from build123d import *

# Parameters (mm, degrees)
CUT_EXTRUDE1_DEPTH       = 5
CUT_EXTRUDE3_DEPTH       = 45
SKETCH8_R                = 40
CUT_EXTRUDE4_DEPTH       = 32
SKETCH9_R                = 32
SKETCH9_R_2              = 24.5
CUT_EXTRUDE5_DEPTH       = 14
SKETCH10_R               = 26
CUT_EXTRUDE6_DEPTH       = 14
FILLET1_R                = 7
FILLET2_R                = 7
CUT_REVOLVE1_START       = 22
CUT_REVOLVE1_DEPTH       = 30.5
CUT_EXTRUDE12_DEPTH      = 5
SKETCH18_W               = 13
SKETCH18_H               = 8
CUT_EXTRUDE13_DEPTH      = 5
INTERSECT1_OUTLINE_R     = 42
INTERSECT1_DEPTH         = 55
SKETCH20_W               = 6
SKETCH20_H               = 3
BOSS_EXTRUDE1_DEPTH      = 8
BOSS_EXTRUDE2_DEPTH      = 1
BOSS_EXTRUDE2_DEPTH_BACK = 1
SKETCH21_W               = 6
SKETCH21_H               = 6
BOSS_EXTRUDE3_DEPTH      = 7
SKETCH19_R               = 1.5
CUT_EXTRUDE14_DEPTH      = 8
SKETCH23_W               = 20
SKETCH23_H               = 7
CUT_EXTRUDE15_DEPTH      = 7
SKETCH24_W               = 44
SKETCH24_H               = 3.5
CUT_EXTRUDE16_DEPTH      = 5


# Read off the part's stored shape, not the designer's step: Cut-Revolve1, Intersect1
with BuildPart() as part:
    # Sketch1 → Revolve1 (revolve)
    with BuildSketch(Plane.XY, mode=Mode.PRIVATE) as revolve1_sk:
        with BuildLine():
            Line((22.5, 0), (32, 0))
            ThreePointArc((32, 0), (33.414213562, 0.585786438), (34, 2))
            Line((34, 2), (34, 18))
            Line((34, 18), (40, 18))
            ThreePointArc((40, 18), (41.414213562, 18.585786438), (42, 20))
            Line((42, 20), (42, 55))
            ThreePointArc((42, 55), (40.535533906, 58.535533906), (37, 60))
            Line((37, 60), (0, 60))
            Line((0, 60), (0, 18))
            Line((0, 18), (22.5, 18))
            Line((22.5, 18), (22.5, 0))
        make_face()
    revolve(revolve1_sk.sketch.rotate(Axis((0, 2, 0), (0, 1, 0)), 90), axis=Axis((0, 2, 0), (0, 1, 0)))

    # Sketch5 → Cut-Extrude1 (cut)
    with BuildSketch(Plane(origin=(0, 60, 0), x_dir=(1, 0, 0), z_dir=(0, 1, 0))):
        with BuildLine():
            Line((-42, 0), (-40, 0))
            Line((-40, 0), (40, 0))
            Line((40, 0), (42, 0))
            ThreePointArc((42, 0), (0, 42), (-42, 0))
        make_face()
    extrude(amount=-CUT_EXTRUDE1_DEPTH, mode=Mode.SUBTRACT)

    # Sketch7 → Cut-Extrude3 (cut)
    with BuildSketch(Plane.XZ.offset(-18)):
        with BuildLine():
            Line((-21, 0), (21, 0))
            ThreePointArc((21, 0), (0, -21), (-21, 0))
        make_face()
    extrude(amount=-CUT_EXTRUDE3_DEPTH, mode=Mode.SUBTRACT)

    # Sketch8 → Cut-Extrude4 (cut)
    with BuildSketch(Plane(origin=(0, 52.5, 0), x_dir=(1, 0, 0), z_dir=(0, 1, 0))):
        with Locations(Location((0, 0, 0), (0, 0, 270))):
            Circle(SKETCH8_R)
        with BuildLine():
            Line((22.912878475, -2), (-22.912878475, -2))
            ThreePointArc((-22.912878475, -2), (0, 23), (22.912878475, -2))
        make_face(mode=Mode.SUBTRACT)
    extrude(amount=-CUT_EXTRUDE4_DEPTH, mode=Mode.SUBTRACT)

    # Sketch9 → Cut-Extrude5 (cut)
    with BuildSketch(Plane(origin=(0, 2, 0), x_dir=(-1, 0, 0), z_dir=(0, -1, 0))):
        with Locations(Location((0, 0, 0), (0, 0, 90))):
            Circle(SKETCH9_R)
        with Locations(Location((0, 0, 0), (0, 0, 90))):
            Circle(SKETCH9_R_2, mode=Mode.SUBTRACT)
    extrude(amount=-CUT_EXTRUDE5_DEPTH, mode=Mode.SUBTRACT)

    # Sketch10 → Cut-Extrude6 (cut)
    with BuildSketch(Plane(origin=(0, 2, 0), x_dir=(-1, 0, 0), z_dir=(0, -1, 0))):
        Circle(SKETCH10_R)
    extrude(amount=-CUT_EXTRUDE6_DEPTH, mode=Mode.SUBTRACT)

    # Fillet1
    fillet1_edges = [part.edges().sort_by_distance(p)[0] for p in [
        (21, 36.5, 0),
        (-21, 36.5, 0),
    ]]
    fillet(fillet1_edges, radius=FILLET1_R)

    # Fillet2
    fillet2_edges = [part.edges().sort_by_distance(p)[0] for p in [
        (-22.912878475, 36.5, 2),
        (22.912878475, 36.5, 2),
    ]]
    fillet(fillet2_edges, radius=FILLET2_R)

    # Cut-Revolve1 outline → Cut-Revolve1 (cut)
    with BuildSketch(Plane(origin=(0, 0, 0), x_dir=(1, 0, 0), z_dir=(0, 1, 0)).offset(CUT_REVOLVE1_START)):
        with BuildLine():
            Line((-34.641016151, -20), (-36.373066959, -21))
            ThreePointArc((-36.373066959, -21), (0, -42), (36.373066959, -21))
            Line((36.373066959, -21), (34.641016151, -20))
            ThreePointArc((34.641016151, -20), (0, -40), (-34.641016151, -20))
        make_face()
    extrude(amount=CUT_REVOLVE1_DEPTH, mode=Mode.SUBTRACT)

    # Sketch15 → Cut-Extrude12 (cut)
    with BuildSketch(Plane(origin=(0, 20.5, 0), x_dir=(1, 0, 0), z_dir=(0, 1, 0))):
        with BuildLine():
            Line((-28.124355653, -3.514579578), (-26.124355653, -3.514579578))
            ThreePointArc((-26.124355653, -3.514579578), (-24.710142091, -2.928793141), (-24.124355653, -1.514579578))
            Line((-24.124355653, -1.514579578), (-24.124355653, 8.485420422))
            ThreePointArc((-24.124355653, 8.485420422), (-24.710142091, 9.899633984), (-26.124355653, 10.485420422))
            Line((-26.124355653, 10.485420422), (-28.124355653, 10.485420422))
            ThreePointArc((-28.124355653, 10.485420422), (-29.538569215, 9.899633984), (-30.124355653, 8.485420422))
            Line((-30.124355653, 8.485420422), (-30.124355653, -1.514579578))
            ThreePointArc((-30.124355653, -1.514579578), (-29.538569215, -2.928793141), (-28.124355653, -3.514579578))
        make_face()
    extrude(amount=-CUT_EXTRUDE12_DEPTH, mode=Mode.SUBTRACT)

    # Sketch18 → Cut-Extrude13 (cut)
    with BuildSketch(Plane(origin=(0, 55, 0), x_dir=(1, 0, 0), z_dir=(0, 1, 0))):
        with Locations((0.796512215, 32.951769165)):
            Rectangle(SKETCH18_W, SKETCH18_H)
    extrude(amount=-CUT_EXTRUDE13_DEPTH, mode=Mode.SUBTRACT)

    # Intersect1 outline → Intersect1 (cut)
    with BuildSketch(Plane(origin=(0, 0, 0), x_dir=(1, 0, 0), z_dir=(0, 1, 0))):
        Circle(INTERSECT1_OUTLINE_R)
        with BuildLine():
            Line((12.124355653, 0), (-12.124355653, 0))
            ThreePointArc((-12.124355653, 0), (-18.186533479, 3.5), (-18.186533479, 10.5))
            ThreePointArc((-18.186533479, 10.5), (0, 21), (18.186533479, 10.5))
            ThreePointArc((18.186533479, 10.5), (18.186533479, 3.5), (12.124355653, 0))
        make_face(mode=Mode.SUBTRACT)
    extrude(amount=INTERSECT1_DEPTH, mode=Mode.SUBTRACT)

    # Sketch20 → Boss-Extrude1 (add)
    with BuildSketch(Plane.XZ.offset(-55)):
        with Locations((0, 33.5)):
            Rectangle(SKETCH20_W, SKETCH20_H)
    extrude(amount=BOSS_EXTRUDE1_DEPTH)

    # Sketch21 → Boss-Extrude2 (add, two sides: drawn at the far end of the back side and taken through both)
    with BuildSketch(Plane.XZ.offset(-47).offset(-BOSS_EXTRUDE2_DEPTH_BACK)):
        with Locations((0, 32)):
            Rectangle(SKETCH21_W, SKETCH21_H)
    extrude(amount=BOSS_EXTRUDE2_DEPTH + BOSS_EXTRUDE2_DEPTH_BACK)

    # Sketch22 → Boss-Extrude3 (add)
    with BuildSketch(Plane(origin=(0, 0, 0), x_dir=(-1, 0, 0), z_dir=(0, 0, -1))):
        with BuildLine():
            Line((-42, 55), (42, 55))
            ThreePointArc((42, 55), (40.535533906, 58.535533906), (37, 60))
            Line((37, 60), (-37, 60))
            ThreePointArc((-37, 60), (-40.535533906, 58.535533906), (-42, 55))
        make_face()
    extrude(amount=BOSS_EXTRUDE3_DEPTH)

    # Sketch19 → Cut-Extrude14 (cut)
    with BuildSketch(Plane(origin=(0, 0, -7), x_dir=(-1, 0, 0), z_dir=(0, 0, -1))):
        with Locations((0, 57.5)):
            Circle(SKETCH19_R)
        with Locations((-30, 57.5)):
            Circle(SKETCH19_R)
        with Locations((30, 57.5)):
            Circle(SKETCH19_R)
    extrude(amount=-CUT_EXTRUDE14_DEPTH, mode=Mode.SUBTRACT)

    # Sketch23 → Cut-Extrude15 (cut)
    with BuildSketch(Plane(origin=(0, 60, 0), x_dir=(1, 0, 0), z_dir=(0, 1, 0))):
        with Locations((-32, 3.5)):
            Rectangle(SKETCH23_W, SKETCH23_H)
        with Locations((32, 3.5)):
            Rectangle(SKETCH23_W, SKETCH23_H)
    extrude(amount=-CUT_EXTRUDE15_DEPTH, mode=Mode.SUBTRACT)

    # Sketch24 → Cut-Extrude16 (cut)
    with BuildSketch(Plane(origin=(0, 60, 0), x_dir=(1, 0, 0), z_dir=(0, 1, 0))):
        with Locations((0, 5.25)):
            Rectangle(SKETCH24_W, SKETCH24_H)
    extrude(amount=-CUT_EXTRUDE16_DEPTH, mode=Mode.SUBTRACT)


solid = part.part
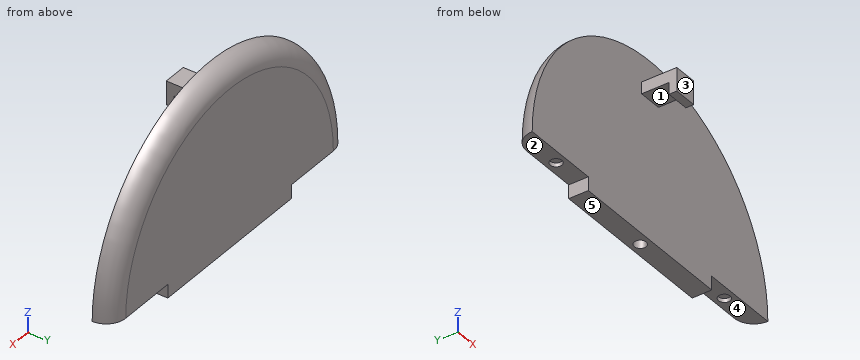
Could you check a few things on this model? Use its own coordinates, in mm. Face numbers are marked on the shaded views. A direction names the side the tool comes from. Coordinates: 2 decimals unless noted, no trailing zeros. Order: outer loops, then holes, each group sorted by start corner. A loop starts at its lowest first (then second) coordinate and runs counter-clockwise, first axis right, second up. Notation, with made-up numbers: (51.25, 73) - (90.25, 73) arc R28 ccw to (90.25, 93) - close; hole circle Ø1 at (75, 38.5). An arc over 180 degrees is marked (long way). Answer in a Markdown table with one row per item. Add a question column.
(1) If we section it at B-B, the plane y = 52.25: Please give me the cut outline in (x, z).
(2) Will these pins go through, and if not, where does the flat tip stop? pin 1 (1.8 mm diameter, centred on y = 52, z = 32, fed in from +X); pin 2 (5.5 mm diameter, centred on x = 28.5, y = 57.5, fed in from -Z); pin 3 (1.5 mm diameter, centred on x = 30, y = 57.5, fed in from -Z).
(3) On a 3-axis mill with a long thin cutter (end or side, diameter ignored), from which of +Z, -Z, +X, -X, +Y, -Y can I reach the whole of each face in a straight line? I mean the marked faces 4 and 5. Say none if no direction works.
(4) If we mould it in two halves opening along Y, with no side actions, what happens to the marked faces 1, 2 and 3? For each: released by +Y, released by -Y, zero draft, split by the parting line, or undercut.
(5) I need wall thicknesses on L1, parallel to Y at x = 0, z = 0; L2, parallel to Z at x = -2.5, y = 51; L3, parallel to Y at x = -0.5, z = 11. Which ranges of each line are inside material? Lowest first, please.
(6) If we section it at A-A, the plane x = 0: Please give me the cut outline in (y, z).
Results are:
| question | item | result |
|---|---|---|
| 1 | outline | (-3, 32) - (3, 32) - (3, 35) - (-3, 35) - close |
| 2 | pin 1 | stops at x = 3 |
| 2 | pin 2 | stops at z = 0 |
| 2 | pin 3 | stops at z = 1 |
| 3 | face 4 | -Z, +X, +Y, -Y |
| 3 | face 5 | -Z, +X, -X, +Y, -Y |
| 4 | face 1 | undercut |
| 4 | face 2 | zero draft |
| 4 | face 3 | released by -Y |
| 5 | L1 | y = 55 to 56, 59 to 60 |
| 5 | L2 | z = 32 to 35 |
| 5 | L3 | y = 55 to 60 |
| 6 | outline | (46, 29) - (48, 29) - (48, 32) - (55, 32) - (55, -3.5) - (56, -3.5) - (56, 1) - (59, 1) - (59, -3.5) - (60, -3.5) - (60, 37) arc R5 ccw to (55, 42) - (55, 35) - (46, 35) - close |
